```python
from build123d import *

# Parameters (mm, degrees)
F3_DEPTH = 120
F6_DEPTH = 10
F7_R     = 3
F8_DEPTH = 30


with BuildPart() as f1:
    # F0 (on Front) → F1 (revolve)
    with BuildSketch(Plane.XZ):
        Polygon((236.6450538874, -62.5779533936), (-663.3549461126, -62.5779533936), (-663.3549461126, -97.5779533936), (396.6450538874, -97.5779533936), (396.6450538874, -65.0779533936), (236.6450538874, -65.0779533936), align=None)
    revolve(axis=Axis((-133.3549461126, 0, -97.5779533936), (-1, 0, 0)))

    # F2 (on face) → F3 (cut)
    with BuildSketch(Plane.YZ.offset(396.6450538874)):
        with BuildLine():
            Line((-21.2289929393, -88.5779533936), (-31.2289929393, -88.5779533936))
            ThreePointArc((-31.2289929393, -88.5779533936), (-32.5, -97.5779533936), (-31.2289929393, -106.5779533936))
            Line((-31.2289929393, -106.5779533936), (-21.2289929393, -106.5779533936))
            Line((-21.2289929393, -106.5779533936), (-21.2289929393, -88.5779533936))
        make_face()
    extrude(amount=-F3_DEPTH, mode=Mode.SUBTRACT)

    # F5 (on offset) → F6 (cut)
    with BuildSketch(Plane.XZ.offset(35)):
        with BuildLine():
            Line((-183.3549461126, -86.1021482944), (-293.3549461126, -86.1021482944))
            ThreePointArc((-293.3549461126, -86.1021482944), (-303.3549461126, -96.1021482944), (-293.3549461126, -106.1021482944))
            Line((-293.3549461126, -106.1021482944), (-183.3549461126, -106.1021482944))
            ThreePointArc((-183.3549461126, -106.1021482944), (-173.3549461126, -96.1021482944), (-183.3549461126, -86.1021482944))
        make_face()
    extrude(amount=-F6_DEPTH, mode=Mode.SUBTRACT)

    # F7 (on face) → F8 (cut)
    with BuildSketch(Plane(origin=(-663.3549461126, 0, 0), x_dir=(0, -1, 0), z_dir=(-1, 0, 0))):
        with Locations((0, -97.5779533936)):
            Circle(F7_R)
    extrude(amount=-F8_DEPTH, mode=Mode.SUBTRACT)


solid = f1.part
```
Build history of the part. All positions in model axes, mm. A direction names the side the tool comes from. Round coordinates to 2 decimals unless told otherwise and drop trailing zeros. Write each loop counter-clockwise with the first axis right and the second up, starting at its lowest first coordinate (ties: lowest second). Pieces come first, ordered by that corner, then holes. Notation, with made-up numbers: (52.5, 20.25) -> (70.5, 20.25) arc R32 cw to (70.5, 55.25) -> close; hole circle Ø2 at (-26.5, -15.75). An arc over 180 degrees is marked (long way). Put each result on its own line as item: value.
Item 1: Slice it at B-B, the plane x = 183. Give the cut face in (y, z).
Here are the results:
outline: circle Ø70 at (0, -97.58)
Item 2: Slice it at A-A, the plane z = -118.5. Give the cut face in (x, y), plus the area to 3 significant figures.
Here are the results:
outline: (-663.35, -28.06) -> (236.65, -28.06) -> (236.65, -24.87) -> (396.65, -24.87) -> (396.65, 24.87) -> (236.65, 24.87) -> (236.65, 28.06) -> (-663.35, 28.06) -> close
area: 58,500 mm^2
Item 3: Two-plate mould, pull along Z, no slides. Class faces 4 (the face through (337, -21.229, -98)), 5 (the face through (315.525, 32.223, -101.809)), 6 (the face through (396.645, 1, -97)): pulls with the +Z half, pulls with the -Z half, needs draft (parallel to the pull), parting line crosses it, or undercut.
Here are the results:
face 4: undercut
face 5: parting line crosses it
face 6: needs draft
Item 4: Tool access for faces 1 (the face through (-239, -25, -96)), 2 (the face through (-219.655, 34.702, -102.134)), 3 (the face through (236.645, -10, -129)): list every direction of +Z, -Z, +X, -X, +Y, -Y with a clear straight run to the whole face (end or side of a thin tool).
Here are the results:
face 1: -Y
face 2: +X, -X
face 3: +X
Item 5: Flat gauge pins, fed straight in: P1, Ø4, axis at x = -462, z = -103.5, coming from the +Y side; P2, Ø10, axis at x = 98.5, y = 6, coming from the +Z side; P3, Ø3, axis at x = 321, y = -26.5, coming from the -Z side. Where does each tip first touch, or does it go through?
Here are the results:
P1: stops at y = 34.78
P2: stops at z = -62.59
P3: stops at z = -118.34
Item 6: Wall check: probe 1 along Y at (x, z) = (-427, -96.5); probe 2 along X at (y, z) = (-22.5, -98); probe 3 along Z at (x, y) = (-550, -3). Give the ranges that are in metal, low to high. Write a range as from..to.
Here are the results:
probe 1: y = -34.98..34.98
probe 2: x = -663.35..276.65
probe 3: z = -132.45..-62.71
